```python
from build123d import *

# Parameters (mm, degrees)
F1_DEPTH     = 1.5
F2_DEPTH     = 20
F4_W         = 26.8
F4_H         = 20.4379309565
F5_DEPTH     = 26
F6_R         = 3
F7_R         = 0.5
F9_DEPTH     = 1.5
F10_W        = 18
F10_H        = 18
F11_DEPTH    = 15
F12_R        = 5
F13_W        = 4.3204394169
F13_H        = 29.8547168866
F14_DEPTH    = 5
F15_R        = 4.99999
F16_W        = 4.3204394169
F16_H        = 4.5489102274
F17_DEPTH    = 5
F18_T1_DEPTH = 29.218490554


# Not quite as in the source:
# - a fillet or chamfer that OpenCascade refuses, or shapes differently, is made with other operations: its cross-section is extruded or revolved along the edge and cut away or added
# - a fillet or chamfer is up to 0.001 mm smaller than in the source, because OpenCascade refuses the exact size


with BuildPart() as f1:
    # F0 (on Top) → F1 (new body)
    with BuildSketch(Plane.XY):
        Polygon((0, -17.6669182372), (15.3, -8.8334591186), (15.3, 8.8334591186), (0, 17.6669182372), (-15.3, 8.8334591186), (-15.3, -8.8334591186), align=None)
        with BuildLine():
            ThreePointArc((-6.0811183182, -8.4852813742), (-8.4852813742, -8.4852813742), (-8.4852813742, -6.0811183182))
            Line((-8.4852813742, -6.0811183182), (-6.6468037432, -4.2426406871))
            ThreePointArc((-6.6468037432, -4.2426406871), (-4.2426406871, -4.2426406871), (-4.2426406871, -6.6468037432))
            Line((-4.2426406871, -6.6468037432), (-6.0811183182, -8.4852813742))
        make_face(mode=Mode.SUBTRACT)
        with BuildLine():
            ThreePointArc((8.4852813742, -6.0811183182), (8.4852813742, -8.4852813742), (6.0811183182, -8.4852813742))
            Line((6.0811183182, -8.4852813742), (4.2426406871, -6.6468037432))
            ThreePointArc((4.2426406871, -6.6468037432), (4.2426406871, -4.2426406871), (6.6468037432, -4.2426406871))
            Line((6.6468037432, -4.2426406871), (8.4852813742, -6.0811183182))
        make_face(mode=Mode.SUBTRACT)
        with BuildLine():
            ThreePointArc((-8.4852813742, 6.0811183182), (-8.4852813742, 8.4852813742), (-6.0811183182, 8.4852813742))
            Line((-6.0811183182, 8.4852813742), (-4.2426406871, 6.6468037432))
            ThreePointArc((-4.2426406871, 6.6468037432), (-4.2426406871, 4.2426406871), (-6.6468037432, 4.2426406871))
            Line((-6.6468037432, 4.2426406871), (-8.4852813742, 6.0811183182))
        make_face(mode=Mode.SUBTRACT)
        with BuildLine():
            Line((4.2426406871, 6.6468037432), (6.0811183182, 8.4852813742))
            ThreePointArc((6.0811183182, 8.4852813742), (8.4852813742, 8.4852813742), (8.4852813742, 6.0811183182))
            Line((8.4852813742, 6.0811183182), (6.6468037432, 4.2426406871))
            ThreePointArc((6.6468037432, 4.2426406871), (4.2426406871, 4.2426406871), (4.2426406871, 6.6468037432))
        make_face(mode=Mode.SUBTRACT)
    extrude(amount=F1_DEPTH)

    # F0 (on Top) → F2 (join)
    with BuildSketch(Plane.XY):
        Polygon((-17.7, 10.2190997647), (-17.7, -10.2190997647), (0, -20.4381995293), (17.7, -10.2190997647), (17.7, 10.2190997647), (0, 20.4381995293), align=None)
        Polygon((15.3, 8.8334591186), (15.3, -8.8334591186), (0, -17.6669182372), (-15.3, -8.8334591186), (-15.3, 8.8334591186), (0, 17.6669182372), align=None, mode=Mode.SUBTRACT)
    extrude(amount=F2_DEPTH)

    # F4 (on offset) → F5 (cut)
    with BuildSketch(Plane.XZ.offset(-25)):
        with Locations((0, 11.7189654782)):
            Rectangle(F4_W, F4_H)
    extrude(amount=F5_DEPTH, mode=Mode.SUBTRACT)

    # F6
    f6_edges = [f1.edges().sort_by_distance(p)[0] for p in [
        (17.7, 10.2191, 10),
        (-17.7, 10.2191, 10),
        (-17.7, -10.2191, 10),
        (0, -20.4382, 10),
        (17.7, -10.2191, 10),
        (15.3, 8.833459, 10.75),
        (15.3, -8.833459, 10.75),
        (0, -17.666918, 10.75),
        (-15.3, -8.833459, 10.75),
        (-15.3, 8.833459, 10.75),
    ]]
    fillet(f6_edges, radius=F6_R)

    # F7
    f7_edges = [f1.edges().sort_by_distance(p)[0] for p in [
        (-13.6, 9.814955, 1.5),
        (0, 20.4382, 0.75),
        (-7.65, -13.250189, 1.5),
        (-14.898076, -8.601408, 1.5),
        (0, -17.202817, 1.5),
        (-15.3, 0, 1.5),
        (7.65, -13.250189, 1.5),
        (-14.898076, 8.601408, 1.5),
        (14.898076, -8.601408, 1.5),
        (15.3, 0, 1.5),
        (14.898076, 8.601408, 1.5),
        (13.6, 9.814955, 1.5),
    ]]
    fillet(f7_edges, radius=F7_R)

    # F8 (on face) → F9 (join)
    with BuildSketch(Plane.XY.offset(1.5)):
        with BuildLine():
            Line((-8.9667634256, 31.0121076152), (-8.9667634256, 15.2612362518))
            Line((-8.9667634256, 15.2612362518), (-0.25, 20.293861962))
            ThreePointArc((-0.25, 20.293861962), (0, 20.3608492601), (0.25, 20.293861962))
            Line((0.25, 20.293861962), (9.0332365744, 15.2228579614))
            Line((9.0332365744, 15.2228579614), (9.0332365744, 31.0121076152))
            Line((9.0332365744, 31.0121076152), (-8.9667634256, 31.0121076152))
        make_face()
    extrude(amount=-F9_DEPTH)

    # F10 (on face) → F11 (join)
    with BuildSketch(Plane(origin=(0, 0, 0), x_dir=(1, 0, 0), z_dir=(0, 0, -1))):
        with Locations((0.0332365744, -22.0121076152)):
            Rectangle(F10_W, F10_H)
    extrude(amount=F11_DEPTH)

    # F12
    f12_edges = [f1.edges().sort_by_distance(p)[0] for p in [
        (9.033237, 22.012108, -15),
        (0.033237, 13.012108, -15),
        (-8.966763, 22.012108, -15),
        (0.033237, 31.012108, -15),
    ]]
    fillet(f12_edges, radius=F12_R)

    # F13 (on face) → F14 (join)
    with BuildSketch(Plane(origin=(0, 0, 0), x_dir=(1, 0, 0), z_dir=(0, 0, -1))):
        with Locations((0.1270717476, 1.9152508281)):
            Rectangle(F13_W, F13_H)
    extrude(amount=F14_DEPTH)

    # F15 (radius 5 in the source; OpenCascade refuses exactly that, so slightly less here)
    f15_edges = [f1.edges().sort_by_distance(p)[0] for p in [
        (0.127072, -16.842609, -5),
    ]]
    fillet(f15_edges, radius=F15_R)

    # F16 (on face) → F17 (join)
    with BuildSketch(Plane(origin=(0, 0, -5), x_dir=(1, 0, 0), z_dir=(0, 0, -1))):
        with Locations((0.1270717476, -10.7376525015)):
            Rectangle(F16_W, F16_H)
    extrude(amount=F17_DEPTH)

    # F18: fillet of radius 5 on 1 edges, made by hand

    # F18_s2 → F18_t1 (cut)
    with BuildSketch(Plane.YZ.offset(-14.4821735295)):
        with BuildLine():
            ThreePointArc((8.4631973878, -5.0203897726), (9.7716225976, -8.3926702426), (13.0121076152, -10))
            Line((13.0121076152, -10), (13.0030858197, -10.0995922045))
            ThreePointArc((13.0030858197, -10.0995922045), (10.7376525015, -10.1), (8.4631973878, -10.1))
            Line((8.4631973878, -10.1), (8.3631973878, -10))
            Line((8.3631973878, -10), (8.3631973878, -5.0203897726))
            Line((8.3631973878, -5.0203897726), (8.4631973878, -5.0203897726))
        make_face()
    extrude(amount=F18_T1_DEPTH, mode=Mode.SUBTRACT)


solid = f1.part
```
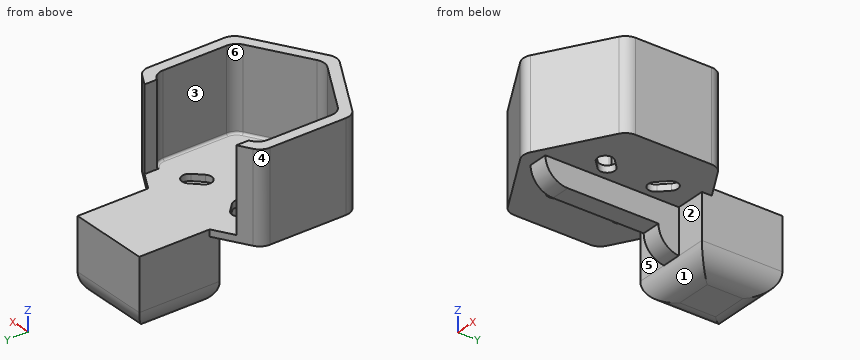
The listing builds one solid part. Answer for the finished solid, in the listing's coordinates (mm). Face numbers are marked on the shaded views. A direction names the side the tool comes from. Give positions to 0.01 mm unless a question says otherwise; leave off trailing zeros. Order: outer loops, then holes, each group sorted by start corner. A loop starts at its lowest first (then second) coordinate and runs counter-clockwise, first axis right, second up. Notation, with made-up numbers: (39, 19.25) - (82, 19.25) arc R34 ccw to (82, 57.25) - close; hole circle Ø3 at (72.25, -17). An arc over 180 degrees is marked (long way). Answer in a Markdown table with one row per item. Add a question column.
Q1. The part is cut by section C-C (y = 3). Determine the outline of the cut face in (x, z).
Q2. For a pull along X with two mould halves and no side action, classify the marked faces 4, 5 and 6 as released by +X, released by -X, zero draft, split by the parting line, or undercut.
Q3. The part is cut by section A-A (z = 9). Determine the outline of the cut face in (x, y), then the cut area to 3 significant figures.
Q4. Find the intervals of material crossed by line 1 along X through (y, z) = (4, 10); line 2 along Y through (x, z) = (8, -2); line 3 along X through (y, z) = (26, -3), in increasing order. Write a range as [from, to].
Q5. Given P1, Ø10, axis at y = -15, z = 7.5, coming from the -X side; P2, Ø1.5, axis at x = 8, z = 14, coming from the +Y side; P3, Ø3, axis at y = -2.5, z = -2.5, coming from the +X side, each flat-ended and moving along its own axis, determine where each tip first touches the part or whether it passes through.
Q6. The part is cut by section D-D (z = -6.5). Determine the outline of the cut face in (x, y), then the cut area to 3 significant figures.
Q7. Which of the six approach directions +Z, -Z, +X, -X, +Y, -Y give full straight-line access (tool end or side, diameter ignored) to the marked faces 1, 2 and 3?
Determined:
| question | item | result |
|---|---|---|
| 1 | outline | (-17.7, 0) - (-2.03, 0) - (-2.03, -5) - (2.29, -5) - (2.29, 0) - (17.7, 0) - (17.7, 20) - (15.3, 20) - (15.3, 2) arc R0.5 cw to (14.8, 1.5) - (-14.8, 1.5) arc R0.5 cw to (-15.3, 2) - (-15.3, 20) - (-17.7, 20) - close |
| 2 | face 4 | released by -X |
| 2 | face 5 | zero draft |
| 2 | face 6 | undercut |
| 3 | outline | (-17.7, -8.49) arc R3 ccw to (-16.2, -11.09) - (-1.5, -19.57) arc R3 ccw to (1.5, -19.57) - (16.2, -11.09) arc R3 ccw to (17.7, -8.49) - (17.7, 8.49) arc R3 ccw to (16.2, 11.09) - (13.4, 12.7) - (13.4, 9.93) - (13.8, 9.7) arc R3 cw to (15.3, 7.1) - (15.3, -7.1) arc R3 cw to (13.8, -9.7) - (1.5, -16.8) arc R3 cw to (-1.5, -16.8) - (-13.8, -9.7) arc R3 cw to (-15.3, -7.1) - (-15.3, 7.1) arc R3 cw to (-13.8, 9.7) - (-13.4, 9.93) - (-13.4, 12.7) - (-16.2, 11.09) arc R3 ccw to (-17.7, 8.49) - close |
| 3 | area | 200 mm² |
| 4 | line 1 | x = [-17.7, -15.3], [15.3, 17.7] |
| 4 | line 2 | y = [13.01, 31.01] |
| 4 | line 3 | x = [-8.97, 9.03] |
| 5 | P1 | stops at x = -17.29 |
| 5 | P2 | stops at y = -12.62 |
| 5 | P3 | stops at x = 2.29 |
| 6 | outline | (-8.97, 13.01) - (-2.03, 13.01) - (-2.03, 8.69) - (2.29, 8.69) - (2.29, 13.01) - (9.03, 13.01) - (9.03, 31.01) - (-8.97, 31.01) - close |
| 6 | area | 343 mm² |
| 7 | face 1 | -Z, +X, -X, -Y |
| 7 | face 2 | -Z, +X, -Y |
| 7 | face 3 | +Z |
